Model file for the job. Use its own axes, mm. A direction names the side the tool comes from. Give positions to 0.01 mm unless a question says otherwise; leave off trailing zeros. Loops run counter-clockwise (first coordinate to the right, second up) from the corner with the lowest first, then second, coordinate; pieces in that order, holes last. Notation, with made-up numbers: (83.5, -36) - (89.5, -36) arc R13 cw to (89.5, -23) - close; hole circle Ø1 at (8.25, 44.5). An arc over 180 degrees is marked (long way). Answer as CSV lines item,"result". Start each with the question number.
Item 1: Pull direction X, two halves, no side cores. Call faces 1 (the cylindrical face through (-42.7, 1.5, 42.4)), 2 (the cylindrical face through (43.64, 1.48, -43.6)), 3 (the flat face through (-1, 3, -1)): pulls with the +X half, pulls with the -X half, needs draft (parallel to the pull), parting line crosses it, or undercut.
Item 2: Tool access for faces 4 (the flat face through (2.5, 1, 11)), 5 (the flat face through (1, 1, -44.5)): list every direction of +Z, -Z, +X, -X, +Y, -Y with a clear straight run to the whole face (end or side of a thin tool).
Item 3: Saw through at A-A on x = -10.5. Give the cut face in (y, z).
Item 4: Drill centre lines: L1, parallel to X at y = 1, z = -41.5; L2, parallel to X at y = 1.5, z = 33.5. Where is each one in solid material? Low to high. Write a range as from..to.
Item 5: Saw through at B-B on y = 2.2. State how many separate pieces and enclosed holes the cut face has, plus the area to 3 significant figures.
from build123d import *

# Parameters (mm, degrees)
SKETCH1_R           = 1.5
BOSS_EXTRUDE1_DEPTH = 3


with BuildPart() as part:
    # Sketch1 → Boss-Extrude1 (new body)
    with BuildSketch(Plane(origin=(0, 0, 0), x_dir=(1, 0, 0), z_dir=(0, 1, 0))):
        with BuildLine():
            Line((-41.5, -44.5), (41.5, -44.5))
            ThreePointArc((41.5, -44.5), (43.621320344, -43.621320344), (44.5, -41.5))
            Line((44.5, -41.5), (44.5, 41.5))
            ThreePointArc((44.5, 41.5), (43.621320344, 43.621320344), (41.5, 44.5))
            Line((41.5, 44.5), (-41.5, 44.5))
            ThreePointArc((-41.5, 44.5), (-43.621320344, 43.621320344), (-44.5, 41.5))
            Line((-44.5, 41.5), (-44.5, -41.5))
            ThreePointArc((-44.5, -41.5), (-43.621320344, -43.621320344), (-41.5, -44.5))
        make_face()
        with Locations((-41.5, 41.5)):
            Circle(SKETCH1_R, mode=Mode.SUBTRACT)
        with Locations((41.5, 41.5)):
            Circle(SKETCH1_R, mode=Mode.SUBTRACT)
        with Locations((41.5, -41.5)):
            Circle(SKETCH1_R, mode=Mode.SUBTRACT)
        with Locations((-41.5, -41.5)):
            Circle(SKETCH1_R, mode=Mode.SUBTRACT)
        with BuildLine():
            Line((26, 23.5), (14, 23.5))
            ThreePointArc((14, 23.5), (13.646446609, 23.646446609), (13.5, 24))
            Line((13.5, 24), (13.5, 38))
            ThreePointArc((13.5, 38), (13.646446609, 38.353553391), (14, 38.5))
            Line((14, 38.5), (26, 38.5))
            ThreePointArc((26, 38.5), (26.353553391, 38.353553391), (26.5, 38))
            Line((26.5, 38), (26.5, 24))
            ThreePointArc((26.5, 24), (26.353553391, 23.646446609), (26, 23.5))
        make_face(mode=Mode.SUBTRACT)
        with BuildLine():
            Line((-16.5, -36), (-16.5, -23))
            ThreePointArc((-16.5, -23), (-16.353553391, -22.646446609), (-16, -22.5))
            Line((-16, -22.5), (-3, -22.5))
            ThreePointArc((-3, -22.5), (-2.646446609, -22.646446609), (-2.5, -23))
            Line((-2.5, -23), (-2.5, -36))
            ThreePointArc((-2.5, -36), (-2.646446609, -36.353553391), (-3, -36.5))
            Line((-3, -36.5), (-16, -36.5))
            ThreePointArc((-16, -36.5), (-16.353553391, -36.353553391), (-16.5, -36))
        make_face(mode=Mode.SUBTRACT)
        with BuildLine():
            Line((-35, -36.5), (-22, -36.5))
            ThreePointArc((-22, -36.5), (-21.646446609, -36.353553391), (-21.5, -36))
            Line((-21.5, -36), (-21.5, -23))
            ThreePointArc((-21.5, -23), (-21.646446609, -22.646446609), (-22, -22.5))
            Line((-22, -22.5), (-35, -22.5))
            ThreePointArc((-35, -22.5), (-35.353553391, -22.646446609), (-35.5, -23))
            Line((-35.5, -23), (-35.5, -36))
            ThreePointArc((-35.5, -36), (-35.353553391, -36.353553391), (-35, -36.5))
        make_face(mode=Mode.SUBTRACT)
        with BuildLine():
            Line((2.5, -36), (2.5, -23))
            ThreePointArc((2.5, -23), (2.646446609, -22.646446609), (3, -22.5))
            Line((3, -22.5), (16, -22.5))
            ThreePointArc((16, -22.5), (16.353553391, -22.646446609), (16.5, -23))
            Line((16.5, -23), (16.5, -36))
            ThreePointArc((16.5, -36), (16.353553391, -36.353553391), (16, -36.5))
            Line((16, -36.5), (3, -36.5))
            ThreePointArc((3, -36.5), (2.646446609, -36.353553391), (2.5, -36))
        make_face(mode=Mode.SUBTRACT)
        with BuildLine():
            Line((21.5, -36), (21.5, -23))
            ThreePointArc((21.5, -23), (21.646446609, -22.646446609), (22, -22.5))
            Line((22, -22.5), (35, -22.5))
            ThreePointArc((35, -22.5), (35.353553391, -22.646446609), (35.5, -23))
            Line((35.5, -23), (35.5, -36))
            ThreePointArc((35.5, -36), (35.353553391, -36.353553391), (35, -36.5))
            Line((35, -36.5), (22, -36.5))
            ThreePointArc((22, -36.5), (21.646446609, -36.353553391), (21.5, -36))
        make_face(mode=Mode.SUBTRACT)
        with BuildLine():
            Line((-16.5, -17), (-16.5, -4))
            ThreePointArc((-16.5, -4), (-16.353553391, -3.646446609), (-16, -3.5))
            Line((-16, -3.5), (-3, -3.5))
            ThreePointArc((-3, -3.5), (-2.646446609, -3.646446609), (-2.5, -4))
            Line((-2.5, -4), (-2.5, -17))
            ThreePointArc((-2.5, -17), (-2.646446609, -17.353553391), (-3, -17.5))
            Line((-3, -17.5), (-16, -17.5))
            ThreePointArc((-16, -17.5), (-16.353553391, -17.353553391), (-16.5, -17))
        make_face(mode=Mode.SUBTRACT)
        with BuildLine():
            Line((2.5, -17), (2.5, -4))
            ThreePointArc((2.5, -4), (2.646446609, -3.646446609), (3, -3.5))
            Line((3, -3.5), (16, -3.5))
            ThreePointArc((16, -3.5), (16.353553391, -3.646446609), (16.5, -4))
            Line((16.5, -4), (16.5, -17))
            ThreePointArc((16.5, -17), (16.353553391, -17.353553391), (16, -17.5))
            Line((16, -17.5), (3, -17.5))
            ThreePointArc((3, -17.5), (2.646446609, -17.353553391), (2.5, -17))
        make_face(mode=Mode.SUBTRACT)
        with BuildLine():
            Line((21.5, -17), (21.5, -4))
            ThreePointArc((21.5, -4), (21.646446609, -3.646446609), (22, -3.5))
            Line((22, -3.5), (35, -3.5))
            ThreePointArc((35, -3.5), (35.353553391, -3.646446609), (35.5, -4))
            Line((35.5, -4), (35.5, -17))
            ThreePointArc((35.5, -17), (35.353553391, -17.353553391), (35, -17.5))
            Line((35, -17.5), (22, -17.5))
            ThreePointArc((22, -17.5), (21.646446609, -17.353553391), (21.5, -17))
        make_face(mode=Mode.SUBTRACT)
        with BuildLine():
            Line((-16.5, 2), (-16.5, 15))
            ThreePointArc((-16.5, 15), (-16.353553391, 15.353553391), (-16, 15.5))
            Line((-16, 15.5), (-3, 15.5))
            ThreePointArc((-3, 15.5), (-2.646446609, 15.353553391), (-2.5, 15))
            Line((-2.5, 15), (-2.5, 2))
            ThreePointArc((-2.5, 2), (-2.646446609, 1.646446609), (-3, 1.5))
            Line((-3, 1.5), (-16, 1.5))
            ThreePointArc((-16, 1.5), (-16.353553391, 1.646446609), (-16.5, 2))
        make_face(mode=Mode.SUBTRACT)
        with BuildLine():
            Line((2.5, 2), (2.5, 15))
            ThreePointArc((2.5, 15), (2.646446609, 15.353553391), (3, 15.5))
            Line((3, 15.5), (16, 15.5))
            ThreePointArc((16, 15.5), (16.353553391, 15.353553391), (16.5, 15))
            Line((16.5, 15), (16.5, 2))
            ThreePointArc((16.5, 2), (16.353553391, 1.646446609), (16, 1.5))
            Line((16, 1.5), (3, 1.5))
            ThreePointArc((3, 1.5), (2.646446609, 1.646446609), (2.5, 2))
        make_face(mode=Mode.SUBTRACT)
        with BuildLine():
            Line((21.5, 2), (21.5, 15))
            ThreePointArc((21.5, 15), (21.646446609, 15.353553391), (22, 15.5))
            Line((22, 15.5), (35, 15.5))
            ThreePointArc((35, 15.5), (35.353553391, 15.353553391), (35.5, 15))
            Line((35.5, 15), (35.5, 2))
            ThreePointArc((35.5, 2), (35.353553391, 1.646446609), (35, 1.5))
            Line((35, 1.5), (22, 1.5))
            ThreePointArc((22, 1.5), (21.646446609, 1.646446609), (21.5, 2))
        make_face(mode=Mode.SUBTRACT)
        with BuildLine():
            Line((-35.5, -17), (-35.5, -4))
            ThreePointArc((-35.5, -4), (-35.353553391, -3.646446609), (-35, -3.5))
            Line((-35, -3.5), (-22, -3.5))
            ThreePointArc((-22, -3.5), (-21.646446609, -3.646446609), (-21.5, -4))
            Line((-21.5, -4), (-21.5, -17))
            ThreePointArc((-21.5, -17), (-21.646446609, -17.353553391), (-22, -17.5))
            Line((-22, -17.5), (-35, -17.5))
            ThreePointArc((-35, -17.5), (-35.353553391, -17.353553391), (-35.5, -17))
        make_face(mode=Mode.SUBTRACT)
        with BuildLine():
            Line((-35.5, 2), (-35.5, 15))
            ThreePointArc((-35.5, 15), (-35.353553391, 15.353553391), (-35, 15.5))
            Line((-35, 15.5), (-22, 15.5))
            ThreePointArc((-22, 15.5), (-21.646446609, 15.353553391), (-21.5, 15))
            Line((-21.5, 15), (-21.5, 2))
            ThreePointArc((-21.5, 2), (-21.646446609, 1.646446609), (-22, 1.5))
            Line((-22, 1.5), (-35, 1.5))
            ThreePointArc((-35, 1.5), (-35.353553391, 1.646446609), (-35.5, 2))
        make_face(mode=Mode.SUBTRACT)
        with BuildLine():
            Line((-26, 38.5), (-14, 38.5))
            ThreePointArc((-14, 38.5), (-13.646446609, 38.353553391), (-13.5, 38))
            Line((-13.5, 38), (-13.5, 24))
            ThreePointArc((-13.5, 24), (-13.646446609, 23.646446609), (-14, 23.5))
            Line((-14, 23.5), (-26, 23.5))
            ThreePointArc((-26, 23.5), (-26.353553391, 23.646446609), (-26.5, 24))
            Line((-26.5, 24), (-26.5, 38))
            ThreePointArc((-26.5, 38), (-26.353553391, 38.353553391), (-26, 38.5))
        make_face(mode=Mode.SUBTRACT)
    extrude(amount=BOSS_EXTRUDE1_DEPTH)


solid = part.part
Responses:
1,face 1,"undercut"
1,face 2,"pulls with the +X half"
1,face 3,"needs draft"
2,face 4,"+Y, -Y"
2,face 5,"-Z, +X, -X, +Y, -Y"
3,outline,"(0, -44.5) - (3, -44.5) - (3, -15.5) - (0, -15.5) - close; (0, -1.5) - (3, -1.5) - (3, 3.5) - (0, 3.5) - close; (0, 17.5) - (3, 17.5) - (3, 22.5) - (0, 22.5) - close; (0, 36.5) - (3, 36.5) - (3, 44.5) - (0, 44.5) - close"
4,L1,"-44.5..-43, -40..40, 43..44.5"
4,L2,"-44.5..-35.5, -21.5..-16.5, -2.5..2.5, 16.5..21.5, 35.5..44.5"
5,separate pieces,"1"
5,enclosed holes,"18"
5,area,"5,150 mm2"
